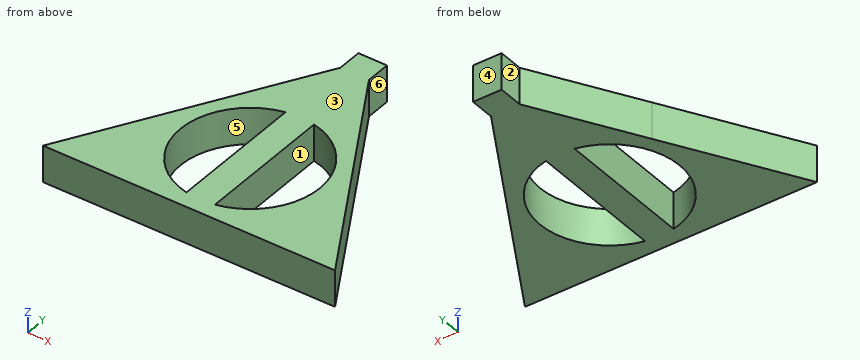
```python
from build123d import *

# Parameters (mm, degrees)
F1_DEPTH = 5


with BuildPart() as f1:
    # F0 (on Top) → F1 (new body)
    with BuildSketch(Plane.XY):
        with BuildLine():
            Line((-1.9610302988, 23.7158841491), (-1.9610302988, 20.3192800363))
            Line((-1.9610302988, 20.3192800363), (-10.0000000112, 6.3953760539))
            ThreePointArc((-10.0000000112, 6.3953760539), (-6.6047488214, 10.093442752), (-1.9610302988, 12.0011393288))
            Line((-1.9610302988, 12.0011393288), (-1.9610302988, 9.9653027286))
            Line((-1.9610302988, 9.9653027286), (-1.9610302988, -8.7215559657))
            Line((-1.9610302988, -8.7215559657), (-1.9610302988, -10.7573925659))
            ThreePointArc((-1.9610302988, -10.7573925659), (-0.9840955869, -10.8831207171), (-3.69e-08, -10.9251320023))
            ThreePointArc((-3.69e-08, -10.9251320023), (0.9840955501, -10.8831207203), (1.9610302988, -10.7573925659))
            Line((1.9610302988, -10.7573925659), (1.9610302988, -8.7215559657))
            Line((1.9610302988, -8.7215559657), (1.9610302988, 9.9653027286))
            Line((1.9610302988, 9.9653027286), (1.9610302988, 12.0011393288))
            ThreePointArc((1.9610302988, 12.0011393288), (6.6047486362, 10.0934428811), (9.9999997855, 6.3953764449))
            Line((9.9999997855, 6.3953764449), (1.9610302988, 20.3192800363))
            Line((1.9610302988, 20.3192800363), (1.9610302988, 23.7158841491))
            Line((1.9610302988, 23.7158841491), (-1.9610302988, 23.7158841491))
        make_face()
        with BuildLine():
            ThreePointArc((-1.9610302988, -10.7573925659), (-10.4556649406, -4.2783719167), (-10.0000000112, 6.3953760539))
            Line((-10.0000000112, 6.3953760539), (-20, -10.9251320023))
            Line((-20, -10.9251320023), (-1.9610302988, -10.9251320023))
            Line((-1.9610302988, -10.9251320023), (-1.9610302988, -10.7573925659))
        make_face()
        with BuildLine():
            ThreePointArc((-1.9610302988, 12.0011393288), (-6.6047488214, 10.093442752), (-10.0000000112, 6.3953760539))
            ThreePointArc((-10.0000000112, 6.3953760539), (-10.4556649406, -4.2783719167), (-1.9610302988, -10.7573925659))
            Line((-1.9610302988, -10.7573925659), (-1.9610302988, -8.7215559657))
            ThreePointArc((-1.9610302988, -8.7215559657), (-9.5470053838, 0.6218733815), (-1.9610302988, 9.9653027286))
            Line((-1.9610302988, 9.9653027286), (-1.9610302988, 12.0011393288))
        make_face()
        with BuildLine():
            ThreePointArc((-3.69e-08, -10.9251320023), (-0.9840955869, -10.8831207171), (-1.9610302988, -10.7573925659))
            Line((-1.9610302988, -10.7573925659), (-1.9610302988, -10.9251320023))
            Line((-1.9610302988, -10.9251320023), (-3.69e-08, -10.9251320023))
        make_face()
        with BuildLine():
            ThreePointArc((1.9610302988, -10.7573925659), (0.9840955501, -10.8831207203), (-3.69e-08, -10.9251320023))
            Line((-3.69e-08, -10.9251320023), (1.9610302988, -10.9251320023))
            Line((1.9610302988, -10.9251320023), (1.9610302988, -10.7573925659))
        make_face()
        with BuildLine():
            Line((1.9610302988, -10.7573925659), (1.9610302988, -10.9251320023))
            Line((1.9610302988, -10.9251320023), (20, -10.9251320023))
            Line((20, -10.9251320023), (9.9999997855, 6.3953764449))
            ThreePointArc((9.9999997855, 6.3953764449), (10.4556650364, -4.2783717123), (1.9610302988, -10.7573925659))
        make_face()
        with BuildLine():
            Line((1.9610302988, -8.7215559657), (1.9610302988, -10.7573925659))
            ThreePointArc((1.9610302988, -10.7573925659), (10.4556650364, -4.2783717123), (9.9999997855, 6.3953764449))
            ThreePointArc((9.9999997855, 6.3953764449), (6.6047486362, 10.0934428811), (1.9610302988, 12.0011393288))
            Line((1.9610302988, 12.0011393288), (1.9610302988, 9.9653027286))
            ThreePointArc((1.9610302988, 9.9653027286), (9.5470053838, 0.6218733815), (1.9610302988, -8.7215559657))
        make_face()
    extrude(amount=F1_DEPTH)


solid = f1.part
```
The listing builds one solid part. Answer for the finished solid, in the listing's coordinates (mm). Face numbers are marked on the shaded views. A direction names the side the tool comes from. Give positions to 0.01 mm unless a question says otherwise; leave off trailing zeros. Write each loop counter-clockwise with the first axis right and the second up, starting at its lowest first coordinate (ties: lowest second). Pieces come first, ordered by that corner, then holes. Notation, with made-up numbers: (31.25, -28.5) - (50.25, -28.5) arc R18 cw to (50.25, 6.5) - close; hole circle Ø3 at (50, -11.75). An arc over 180 degrees is marked (long way). Use one line per item in the form item = value. Start each with the question number.
1) Find section D-D on x = -2.5. Determine the outline of the cut face in (y, z), plus the area to 3 significant figures.
2) Find section C-C on y = 1. Determine the outline of the cut face in (x, z).
3) Consider line 1 along X through (y, z) = (-4, 2); line 2 along X through (y, z) = (-4.5, 0.9); line 3 along Y through (x, z) = (5.5, 2.1). Determine where each line is inside the solid, lowest interval first. Write a range as from..to.
4) A tool of negligible diameter and unlimited length cuts with its end or side. For the marked faces 1, 2 and 3, from which of +Z, -Z, +X, -X, +Y, -Y can it reach the whole face along a straight path? Write none if from no direction.
5) Find section B-B on z = 2.5. Determine the outline of the cut face in (x, y), plus the area to 3 significant figures.
6) Flat-ended cylindrical pins translate along their axes: pin 1 Ø1.5 at (y, z) = (4.5, 2) entering from +X; pin 2 Ø1.7 at (y, z) = (21.5, 3) entering from +X; pin 3 Ø2.5 at (y, z) = (22, 3) entering from -X. Find the tip coordinate at first contact, or state that the pin passes through.
7) The mould has two halves that part along X. Classify the marked faces 4, 5 and 6: pulls with the +X half, pulls with the -X half, needs draft (parallel to the pull), parting line crosses it, or undercut.
8) Find section A-A on x = 3.5. Determine the outline of the cut face in (y, z).
Geometry results:
q1.outline = (-10.93, 0) - (-8.59, 0) - (-8.59, 5) - (-10.93, 5) - close; (9.84, 0) - (19.39, 0) - (19.39, 5) - (9.84, 5) - close
q1.area = 59.4 mm2
q2.outline = (-13.12, 0) - (-9.54, 0) - (-9.54, 5) - (-13.12, 5) - close; (-1.96, 0) - (1.96, 0) - (1.96, 5) - (-1.96, 5) - close; (9.54, 0) - (13.12, 0) - (13.12, 5) - (9.54, 5) - close
q3.line_1 = -16..-8.35, -1.96..1.96, 8.35..16
q3.line_2 = -16.29..-8.06, -1.96..1.96, 8.06..16.29
q3.line_3 = -10.93..-7.18, 8.43..14.19
q4.face_1 = +Z, -Z
q4.face_2 = +Z, -Z, -X, +Y
q4.face_3 = +Z, +X, -X, +Y, -Y
q5.outline = (-20, -10.93) - (20, -10.93) - (1.96, 20.32) - (1.96, 23.72) - (-1.96, 23.72) - (-1.96, 20.32) - close; hole (-1.96, -8.72) - (-1.96, 9.97) arc R9.55 ccw to start; hole (1.96, -8.72) arc R9.55 ccw to (1.96, 9.97) - close
q5.area = 487 mm2
q6.pin_1 = 11.53
q6.pin_2 = 1.96
q6.pin_3 = -1.96
q7.face_4 = needs draft
q7.face_5 = undercut
q7.face_6 = pulls with the +X half
q8.outline = (-10.93, 0) - (-8.26, 0) - (-8.26, 5) - (-10.93, 5) - close; (9.5, 0) - (17.65, 0) - (17.65, 5) - (9.5, 5) - close
